Here's how the part is built. I have some questions about the finished solid (model axes, mm). A direction names the side the tool comes from. Coordinates: 2 decimals unless noted, no trailing zeros. Loops run counter-clockwise (first coordinate to the right, second up) from the corner with the lowest first, then second, coordinate; pieces in that order, holes last. Notation, with made-up numbers: (31.25, 25.25) -> (55.25, 25.25) arc R13 ccw to (55.25, 38.25) -> close; hole circle Ø10 at (84, 10.25). An arc over 180 degrees is marked (long way). Answer as a JSON object with one key per item and string values. Group by question number.
Q1. Thinking about a two-plate mould opening in Y: for faces 1 (the flat face through (0, 25, 11.4)), 2 (the flat face through (-0.1, 25, 1.5)), 3 (the flat face through (0, 30, 12)), which applies, released by +Y, released by -Y, zero draft, split by the parting line, or undercut?
Q2. I need wall thicknesses on line 1 (Y direction, x = 0, z = 1.85); line 2 (Y direction, x = 0, z = 2.1); line 3 (Z direction, x = -4, y = 30.5). Which ranges of each line are inside material? Lowest first, please.
Q3. I want a section at A-A on z = 3.75. Write out the boundary of the cut face in (x, y).
Q4. I want a section at B-B on x = 2.5. Write out the boundary of the cut face in (y, z), then the cut area to 3 significant figures.
Q5. I want a section at C-C on z = 1.5. Write out the boundary of the cut face in (x, y), then the cut area to 3 significant figures.
Q6. I want a section at D-D on y = 26. Write out the boundary of the cut face in (x, z), then the cut area to 3 significant figures.
Q7. On a 3-axis mill with a long thin cutter (end or side, diameter ignored), from which of +Z, -Z, +X, -X, +Y, -Y can I reach the whole of each face in a straight line? I mean faces 4 (the flat face through (4, 4, 6)), 5 (the flat face through (0, 30, 11)), 6 (the cylindrical face through (1.301, -5.857, 3.625)), 7 (the flat face through (0, 30, 1)). Say none if no direction works.
Q8. I'm going to push flat-ended pins straight in: pin 1 (1 mm diameter, centred on y = 4.5, z = 6, fed in from -X); pin 2 (1 mm diameter, centred on x = 2, z = 3, fed in from -Y); pin 3 (4 mm diameter, centred on x = -5, z = 4, fed in from -Y). Where does each tip first touch, or does it pass through?
```python
from build123d import *

# Parameters (mm, degrees)
EXTRUDE_1_DEPTH     = 2
SKETCH_4_R          = 6
SKETCH_4_R_2        = 5
EXTRUDE_2_DEPTH     = 6
SKETCH_5_W          = 12
SKETCH_5_H          = 12
EXTRUDE_3_DEPTH     = 10
CUT_EXTRUDE_1_DEPTH = 10


with BuildPart() as part:
    # 草图1 → 凸台-拉伸1 (new body)
    with BuildSketch(Plane.XY):
        with BuildLine():
            ThreePointArc((-6, 0), (0, 6), (6, 0))
            Line((6, 0), (6, 25))
            Line((6, 25), (-6, 25))
            Line((-6, 25), (-6, 0))
        make_face()
    extrude(amount=EXTRUDE_1_DEPTH)

    # 草图4 → 凸台-拉伸2 (add)
    with BuildSketch(Plane(origin=(0, 0, 0), x_dir=(-1, 0, 0), z_dir=(0, 0, -1))):
        Circle(SKETCH_4_R)
        Circle(SKETCH_4_R_2, mode=Mode.SUBTRACT)
    extrude(amount=-EXTRUDE_2_DEPTH)

    # 草图5 → 凸台-拉伸3 (add)
    with BuildSketch(Plane(origin=(0, 25, 0), x_dir=(1, 0, 0), z_dir=(0, 1, 0))):
        with Locations((0, -6)):
            Rectangle(SKETCH_5_W, SKETCH_5_H)
    extrude(amount=EXTRUDE_3_DEPTH)

    # 草图6 → 切除-拉伸1 (cut)
    with BuildSketch(Plane(origin=(0, 35, 0), x_dir=(1, 0, 0), z_dir=(0, 1, 0))):
        Polygon((5, -1), (-5, -1), (5, -11), align=None)
        Polygon((5, -11), (-5, -1), (-5, -11), align=None)
    extrude(amount=-CUT_EXTRUDE_1_DEPTH, mode=Mode.SUBTRACT)


solid = part.part
```
Result set:
{
 "1": {"face 1": "undercut", "face 2": "released by +Y", "face 3": "zero draft"},
 "2": {"line 1": "y = -6 to -5, 5 to 25", "line 2": "y = -6 to -5, 5 to 6", "line 3": "z = 0 to 1, 11 to 12"},
 "3": {"outline": "circle Ø12 at (0, 0); (-6, 25) -> (-5, 25) -> (-5, 35) -> (-6, 35) -> close; (5, 25) -> (6, 25) -> (6, 35) -> (5, 35) -> close; hole circle Ø10 at (0, 0)"},
 "4": {"outline": "(-5.45, 0) -> (-4.33, 0) -> (-4.33, 6) -> (-5.45, 6) -> close; (4.33, 0) -> (35, 0) -> (35, 1) -> (25, 1) -> (25, 2) -> (5.45, 2) -> (5.45, 6) -> (4.33, 6) -> close; (25, 11) -> (35, 11) -> (35, 12) -> (25, 12) -> close", "area": "72.6 mm²"},
 "5": {"outline": "(-6, 0) arc R6 ccw to (6, 0) -> (6, 35) -> (5, 35) -> (5, 25) -> (-5, 25) -> (-5, 35) -> (-6, 35) -> close; hole circle Ø10 at (0, 0)", "area": "298 mm²"},
 "6": {"outline": "(-6, 0) -> (6, 0) -> (6, 12) -> (-6, 12) -> close; hole (-5, 1) -> (5, 1) -> (5, 11) -> (-5, 11) -> close", "area": "44.0 mm²"},
 "7": {"face 4": "+Z, +X, -X, -Y", "face 5": "+Y, -Y", "face 6": "+Z", "face 7": "+Y"},
 "8": {"pin 1": "stops at x = -4.47", "pin 2": "stops at y = -5.81", "pin 3": "stops at y = -5.2"}
}
